Here's how the part is built. I have some questions about the finished solid (model axes, mm). Face numbers are marked on the shaded views. Give positions to 0.01 mm unless a question says otherwise; leave off trailing zeros. Loops run counter-clockwise (first coordinate to the right, second up) from the corner with the lowest first, then second, coordinate; pieces in that order, holes last. Notation, with made-up numbers: M 29,64 L 49,64 A14 ccw 49,81 Z; hole C -12.75,-26 d6. An arc over 180 degrees is marked long. Answer as CSV lines item,"result". Start each with the question number.
Item 1: I want a section at D-D on x = -19.5. List the corners of the cut face in (y, z) for me, plus the area to 3 significant figures.
Item 2: I want a section at B-B on y = 7. List the corners of the cut face in (x, z) for me, plus the area to 3 significant figures.
Item 3: Will these pins go through, and if not, where does the flat tip stop? P1, Ø2, axis at x = 10.5, z = 1, coming from the -Y side; P2, Ø1.5, axis at x = 7.5, z = 8.5, coming from the +Y side.
Item 4: If we mould it in two halves opening along X, with no side actions, what happens to the marked faces 1, 2 and 3? For each: released by +X, released by -X, zero draft, split by the parting line, or undercut.
Item 5: I want a section at C-C on z = 2.5. List the corners of the cut face in (x, y) for me.
Item 6: If I drill on line 1 along Y through (x, z) = (0, 7.75); line 2 along X through (y, z) = (-1, 0.5); line 3 along X through (y, z) = (-8, 8.5), over which ranges is the centre line in solid material (lowest first)? Write a range as from..to.
Item 7: I want a section at A-A on x = 0. List the corners of the cut face in (y, z) for me.
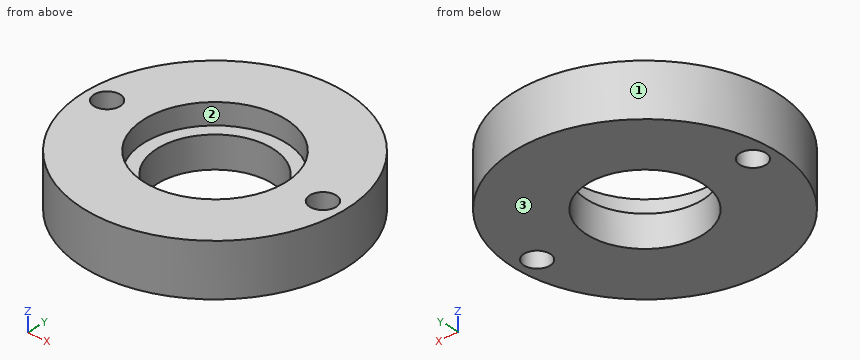
from build123d import *

# Parameters (mm, degrees)
SKETCH_1_R          = 25
EXTRUDE_1_DEPTH     = 10
SKETCH_2_R          = 13.5
CUT_EXTRUDE_1_DEPTH = 4
SKETCH_4_R          = 11
CUT_EXTRUDE_2_DEPTH = 37.742346142
M6X1_0_1_D          = 5


with BuildPart() as part:
    # ｽｹｯﾁ1 → ﾎﾞｽ - 押し出し1 (new body)
    with BuildSketch(Plane.XY):
        Circle(SKETCH_1_R)
    extrude(amount=EXTRUDE_1_DEPTH)

    # ｽｹｯﾁ2 → ｶｯﾄ - 押し出し1 (cut)
    with BuildSketch(Plane.XY.offset(10)):
        Circle(SKETCH_2_R)
    extrude(amount=-CUT_EXTRUDE_1_DEPTH, mode=Mode.SUBTRACT)

    # ｽｹｯﾁ4 → ｶｯﾄ - 押し出し2 (cut, through all)
    with BuildSketch(Plane(origin=(0, 0, 0), x_dir=(-1, 0, 0), z_dir=(0, 0, -1))):
        Circle(SKETCH_4_R)
    extrude(amount=-CUT_EXTRUDE_2_DEPTH, mode=Mode.SUBTRACT)

    # M6x1.0 ねじ穴1 (through all)
    with Locations(Plane(origin=(-21, 0, 10), x_dir=(1, 0, 0), z_dir=(0, 0, 1))):
        with Locations((0, 0), (42, 0)):
            Hole(M6X1_0_1_D / 2)


solid = part.part
Result:
1,outline,"M -15.64,0 L -2,0 L -2,10 L -15.64,10 Z; M 2,0 L 15.64,0 L 15.64,10 L 2,10 Z"
1,area,"273 mm^2"
2,outline,"M -24,0 L -8.49,0 L -8.49,6 L -11.54,6 L -11.54,10 L -24,10 Z; M 8.49,0 L 24,0 L 24,10 L 11.54,10 L 11.54,6 L 8.49,6 Z"
2,area,"286 mm^2"
3,P1,"y = -23.12"
3,P2,"y = 24.07"
4,face 1,"split by the parting line"
4,face 2,"undercut"
4,face 3,"zero draft"
5,outline,"C 0,0 d50; hole C -21,0 d5; hole C 0,0 d22; hole C 21,0 d5"
6,line 1,"-25..-13.5, 13.5..25"
6,line 2,"-24.98..-23.29, -18.71..-10.95, 10.95..18.71, 23.29..24.98"
6,line 3,"-23.69..-10.87, 10.87..23.69"
7,outline,"M -25,0 L -11,0 L -11,6 L -13.5,6 L -13.5,10 L -25,10 Z; M 11,0 L 25,0 L 25,10 L 13.5,10 L 13.5,6 L 11,6 Z"
